```python
from build123d import *

# Parameters (mm, degrees)
SKETCH1_W           = 26.67
SKETCH1_H           = 9.525
SKETCH2_R           = 8.89
BOSS_EXTRUDE1_DEPTH = 0.635
CUT_EXTRUDE1_DEPTH  = 11.16
CHAMFER1_SIZE       = 0.381


with BuildPart() as part:
    # Sketch1 → Revolve1 (revolve)
    with BuildSketch(Plane(origin=(0, 0, 0), x_dir=(-1, 0, 0), z_dir=(0, 0, -1))):
        with Locations((-13.335, -5.3975)):
            Rectangle(SKETCH1_W, SKETCH1_H)
    revolve(axis=Axis((0, -10.16, 0), (0, 1, 0)))

    # Sketch2 → Boss-Extrude1 (add)
    with BuildSketch(Plane(origin=(0, -0.635, 0), x_dir=(-1, 0, 0), z_dir=(0, 1, 0))):
        Circle(SKETCH2_R)
    extrude(amount=BOSS_EXTRUDE1_DEPTH)

    # Sketch3 → Cut-Extrude1 (cut, through all)
    with BuildSketch(Plane.XZ.offset(10.16)):
        Polygon((-7.332348419, 0), (-3.666174209, -6.35), (3.666174209, -6.35), (7.332348419, 0), (3.666174209, 6.35), (-3.666174209, 6.35), align=None)
    extrude(amount=-CUT_EXTRUDE1_DEPTH, mode=Mode.SUBTRACT)

    # Chamfer1
    chamfer1_edges = [part.edges().sort_by_distance(p)[0] for p in [
        (-26.67, -0.635, 0),
        (-26.67, -10.16, 0),
    ]]
    chamfer(chamfer1_edges, length=CHAMFER1_SIZE)


solid = part.part
```
Geometry: final body of the model. Coordinates: model frame, mm. A direction names the side the tool comes from. Round coordinates to 2 decimals unless told otherwise and drop trailing zeros. Order: outer loops, then holes, each group sorted by start corner. A loop starts at its lowest first (then second) coordinate and runs counter-clockwise, first axis right, second up. Notation, with made-up numbers: M -34.5,-19 L -16.5,-19 A16 cw -16.5,-10 Z; hole C 46.5,15 d3. An arc over 180 degrees is marked long. One line per item, written item: value.
(1) Reachability of faces 5 (the flat face through (5, -10.16, 5)), 6 (the flat face through (5.525, -5.151, 3.131)) from +Z, -Z, +X, -X, +Y, -Y: full face, straight path, thin tool, end or side. Return the list, or none.
Result sheet:
face 5: +Z, -Z, +X, -X, -Y
face 6: +Y, -Y
(2) Line query: probe 1 along Y at (x, z) = (12, -23) (3 decimals); probe 2 along Z at (x, y) = (6, -3.5); probe 3 along Z at (x, y) = (5.5, -8). Output: solid intervals per line, ascending. Write a range as [from, to].
Result sheet:
probe 1: [-10.16, -0.635]
probe 2: [-25.99, -2.31], [2.31, 25.99]
probe 3: [-26.1, -3.17], [3.17, 26.1]
(3) Pin query (flat end, axial travel): P1, Ø1, axis at x = -20.5, y = -2, coming from the -Z side; P2, Ø1.5, axis at x = 21, z = -20.5, coming from the -Y side; P3, Ø3, axis at x = -3, y = -4.5, coming from the +Z side; P4, Ø3.5, axis at x = 1, y = -3, coming from the +Z side. Return the tip coordinate at first contact, or that it passes through.
Result sheet:
P1: z = -17.64
P2: through
P3: z = 26.63
P4: z = 26.67
(4) Cut plane A-A (x = 0). Return the cut outline in (y, z) (3 decimals).
Result sheet:
outline: M -10.16,-26.289 L -9.779,-26.67 L -1.016,-26.67 L -0.635,-26.289 L -0.635,-8.89 L 0,-8.89 L 0,-6.35 L -10.16,-6.35 Z; M -10.16,6.35 L 0,6.35 L 0,8.89 L -0.635,8.89 L -0.635,26.289 L -1.016,26.67 L -9.779,26.67 L -10.16,26.289 Z
(5) Pull-direction query (X, two-part tool) for faces 1 (the flat face through (-5.525, -5.151, -3.131)), 2 (the flat face through (11, -0.635, 0)), 3 (the flat face through (-5.474, -5.151, 3.219)), 4 (the cylindrical face through (1.93, -0.32, -8.68)); classes: pulls with the +X half, pulls with the -X half, needs draft (parallel to the pull), parting line crosses it, or undercut.
Result sheet:
face 1: undercut
face 2: needs draft
face 3: undercut
face 4: parting line crosses it
(6) Cut plane B-B (y = -8). Return the cut outline in (x, z).
Result sheet:
outline: C 0,0 d53.34; hole M -7.33,0 L -3.67,-6.35 L 3.67,-6.35 L 7.33,0 L 3.67,6.35 L -3.67,6.35 Z
